Model file for the job. Use its own axes, mm. Face numbers are marked on the shaded views. Round coordinates to 2 decimals unless told otherwise and drop trailing zeros. Order: outer loops, then holes, each group sorted by start corner. A loop starts at its lowest first (then second) coordinate and runs counter-clockwise, first axis right, second up. Notation, with made-up numbers: (72.5, 33) - (113.5, 33) arc R20 ccw to (113.5, 58) - close; hole circle Ø6 at (-32, -24). An arc over 180 degrees is marked (long way). Answer as CSV lines item,"result". Start each with the question number.
1. Pull direction Y, two halves, no side cores. Call the marked faces 1, 2, 3 and 4: released by +Y, released by -Y, zero draft, split by the parting line, or undercut.
2. Band-saw the part on C-C on x = -7.75. List the corners of the cut face in (y, z) (3 decimals), then the cut area to 3 significant figures.
3. Band-saw the part on B-B on x = -15.5. List the corners of the cut face in (y, z) (3 decimals).
4. Band-saw the part on D-D on y = -3.5. List the corners of the cut face in (x, z) (3 decimals), then the cut area to 3 significant figures.
5. Band-saw the part on A-A on y = -12.5. List the corners of the cut face in (x, z) (3 decimals), then the cut area to 3 significant figures.
6. Pin check, flat tips, straight feed: pin 1 Ø3.5 at (x, y) = (7.75, 13.42) entering from +Z (3 decimals); pin 2 Ø1.5 at (y, z) = (0, 1) entering from +X; pin 3 Ø2.5 at (x, y) = (-7.75, 13.42) entering from +Z. Stop position of each tip, or through.
7. Wall check: line 1 along X through (y, z) = (11, 1.05); line 2 along Y through (x, z) = (-7.75, 1.4); line 3 along X through (y, z) = (-14, 0.45). Give the ranges that are in metal, low to high. Write a range as [from, to].
```python
from build123d import *

# Parameters (mm, degrees)
SKETCH1_R                 = 6
BOSS_EXTRUDE1_DEPTH       = 3.175
M3_CLEARANCE_HOLE1_D      = 3.2
FILLET1_R                 = 6.35
F_4_CLEARANCE_HOLE1_D     = 2.9464
F_4_CLEARANCE_HOLE1_DEPTH = 3.302
F_4_CLEARANCE_HOLE1_TIP   = 0.885187864


with BuildPart() as part:
    # Sketch1 → Boss-Extrude1 (new body)
    with BuildSketch(Plane.XY):
        Polygon((-31.498891971, 18.185893759), (0, -36.371787517), (31.498891971, 18.185893759), align=None)
        with Locations((-6.062177826, -3.5)):
            Circle(SKETCH1_R, mode=Mode.SUBTRACT)
    extrude(amount=BOSS_EXTRUDE1_DEPTH)

    # M3 Clearance Hole1 (through all)
    with Locations(Plane(origin=(-27.388360069, 15.242769311, 3.175), x_dir=(1, 0, 0), z_dir=(0, 0, 1))):
        with Locations((19.638360069, -1.819375553), (35.138360069, -1.819375553), (42.888360069, -15.242769311), (11.888360069, -15.242769311), (19.638360069, -28.66616307), (35.138360069, -28.66616307)):
            Hole(M3_CLEARANCE_HOLE1_D / 2)

    # Fillet1
    fillet1_edges = [part.edges().sort_by_distance(p)[0] for p in [
        (31.498891971, 18.185893759, 1.5875),
        (0, -36.371787517, 1.5875),
        (-31.498891971, 18.185893759, 1.5875),
    ]]
    fillet(fillet1_edges, radius=FILLET1_R)

    # #4 Clearance Hole1
    with Locations(Plane(origin=(-21.085137788, 23.004512958, 3.175), x_dir=(1, 0, 0), z_dir=(0, 0, 1))):
        with Locations((0.584768445, -11.1686192), (41.585507131, -11.1686192), (21.085137788, -46.676300475)):
            Hole(F_4_CLEARANCE_HOLE1_D / 2, depth=F_4_CLEARANCE_HOLE1_DEPTH)
            with Locations((0, 0, -(F_4_CLEARANCE_HOLE1_DEPTH + F_4_CLEARANCE_HOLE1_TIP / 2))):  # 118° drill point
                Cone(0, F_4_CLEARANCE_HOLE1_D / 2, F_4_CLEARANCE_HOLE1_TIP, mode=Mode.SUBTRACT)


solid = part.part
```
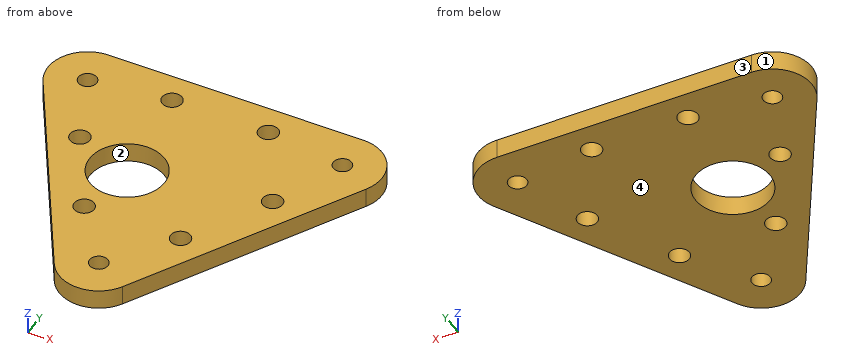
Reply:
1,face 1,"split by the parting line"
1,face 2,"undercut"
1,face 3,"released by +Y"
1,face 4,"zero draft"
2,outline,"(-22.948, 0) - (-15.023, 0) - (-15.023, 3.175) - (-22.948, 3.175) - close; (-11.823, 0) - (-9.258, 0) - (-9.258, 3.175) - (-11.823, 3.175) - close; (2.258, 0) - (11.823, 0) - (11.823, 3.175) - (2.258, 3.175) - close; (15.023, 0) - (18.186, 0) - (18.186, 3.175) - (15.023, 3.175) - close"
2,area,"73.7 mm2"
3,outline,"(-9.525, 0) - (-1.6, 0) - (-1.6, 3.175) - (-9.525, 3.175) - close; (1.6, 0) - (18.186, 0) - (18.186, 3.175) - (1.6, 3.175) - close"
4,outline,"(-18.979, 0) - (-12.062, 0) - (-12.062, 3.175) - (-18.979, 3.175) - close; (-0.062, 0) - (18.979, 0) - (18.979, 3.175) - (-0.062, 3.175) - close"
4,area,"82.4 mm2"
5,outline,"(-13.782, 0) - (-9.057, 0) - (-9.057, 3.175) - (-13.782, 3.175) - close; (-6.443, 0) - (6.443, 0) - (6.443, 3.175) - (-6.443, 3.175) - close; (9.057, 0) - (13.782, 0) - (13.782, 3.175) - (9.057, 3.175) - close"
5,area,"70.9 mm2"
6,pin 1,"stops at z = 3.175"
6,pin 2,"stops at x = 21.43"
6,pin 3,"passes through"
7,line 1,"x = [-26.8, -21.71], [-19.29, 19.29], [21.71, 26.8]"
7,line 2,"y = [-22.95, -15.02], [-11.82, -9.26], [2.26, 11.82], [15.02, 18.19]"
7,line 3,"x = [-12.92, -9.24], [-6.26, 6.26], [9.24, 12.92]"
